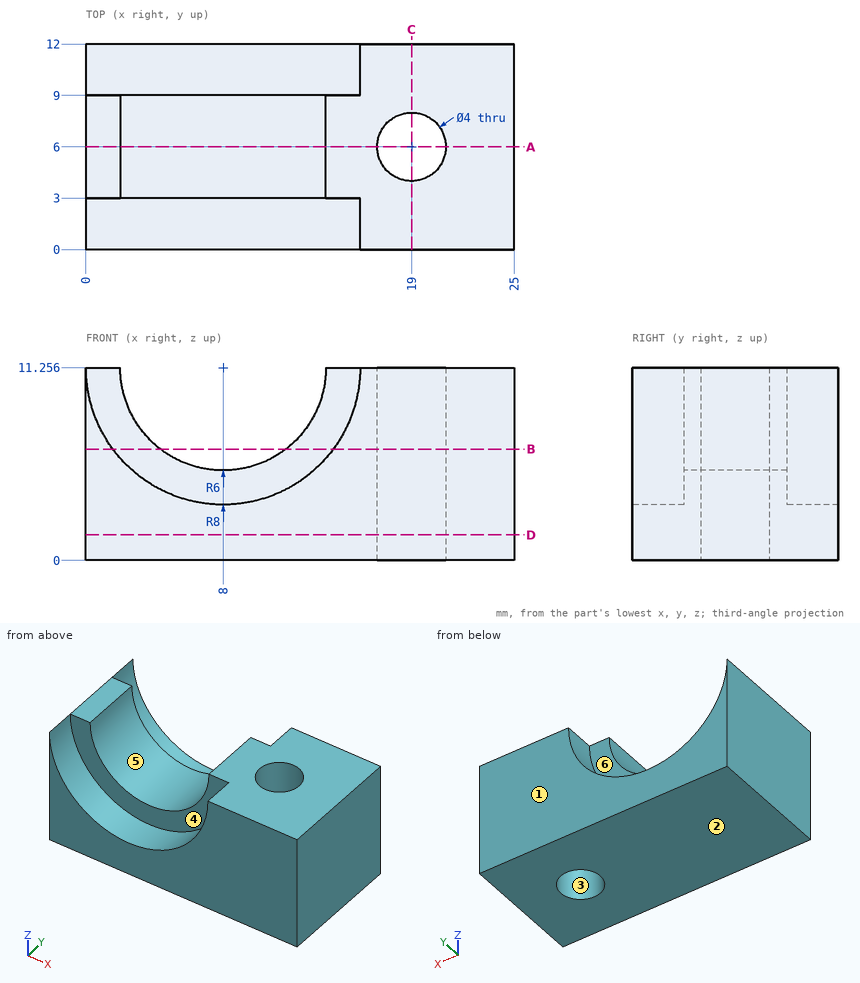
Could you check a few things on this drawing? It's one solid part, dimensions in mm from its lowest x, y, z. A direction names the side the tool comes from. Coordinates: 2 decimals unless noted, no trailing zeros. Write each loop counter-clockwise with the first axis right and the second up, starting at its lowest first coordinate (ties: lowest second). Pieces come first, ordered by that corner, then holes. Notation, with made-up numbers: M 75.5,78 L 94.5,78 A22 ccw 94.5,96 Z; hole C 13,-7.75 d8. An arc over 180 degrees is marked long. Answer as CSV lines item,"result". Start each with the question number.
Q1. Will these pins go through, and if not, where does the flat tip stop? pin 1 Ø2.5 at (x, z) = (7.5, 5.5) entering from +Y; pin 2 Ø1.5 at (x, z) = (13, 7) entering from -Y.
Q2. I need wall thicknesses on probe 1 along Y at (x, z) = (19, 7.5); probe 2 along X at (y, z) = (9.5, 5) (1 decimal); probe 3 along Y at (x, z) = (3.25, 6). Which ranges of each line are inside material? Lowest first, please. Write a range as [from, to].
Q3. Suppose I cut it at B-B, the plane z = 6.5. List the corners of the cut face in (x, y) for me.
Q4. If we mould it in two halves opening along Y, with no side actions, what happens to the marked faces 1, 2 and 3? For each: pulls with the +Y half, pulls with the -Y half, needs draft (parallel to the pull), parting line crosses it, or undercut.
Q5. For the marked faces 4, 5 and 6, which set-ups out of +Z, -Z, +X, -X, +Y, -Y let a thin tool reach every point of the face, with its end or its side?
Q6. Suppose I cut it at D-D, the plane z = 1.5. List the corners of the cut face in (x, y) for me.
Q7. Suppose I cut it at A-A, the plane y = 6. List the corners of the cut face in (x, z) for me, then the cut area to 3 significant figures.
Q8. Suppose I cut it at C-C, the plane x = 19. List the corners of the cut face in (y, z) for me.
Entries:
1,pin 1,"stops at y = 9"
1,pin 2,"stops at y = 3"
2,probe 1,"y = [0, 4], [8, 12]"
2,probe 2,"x = [0, 3], [13, 25]"
2,probe 3,"y = [3, 9]"
3,outline,"M 0,0 L 1.57,0 L 1.57,3 L 4.34,3 L 4.34,9 L 1.57,9 L 1.57,12 L 0,12 Z; M 11.66,3 L 14.43,3 L 14.43,0 L 25,0 L 25,12 L 14.43,12 L 14.43,9 L 11.66,9 Z; hole C 19,6 d4"
4,face 1,"pulls with the +Y half"
4,face 2,"needs draft"
4,face 3,"undercut"
5,face 4,"+Z, -Y"
5,face 5,"+Z, +Y, -Y"
5,face 6,"+Z, +Y"
6,outline,"M 0,0 L 25,0 L 25,12 L 0,12 Z; hole C 19,6 d4"
7,outline,"M 0,0 L 17,0 L 17,11.26 L 14,11.26 A6 cw 2,11.26 L 0,11.26 Z; M 21,0 L 25,0 L 25,11.26 L 21,11.26 Z"
7,area,"180 mm²"
8,outline,"M 0,0 L 4,0 L 4,11.26 L 0,11.26 Z; M 8,0 L 12,0 L 12,11.26 L 8,11.26 Z"
